Build history of the part. All positions in model axes, mm. Give positions to 0.01 mm unless a question says otherwise; leave off trailing zeros. Order: outer loops, then holes, each group sorted by start corner. A loop starts at its lowest first (then second) coordinate and runs counter-clockwise, first axis right, second up. Notation, with made-up numbers: (-17.5, 28.25) - (-2.5, 28.25) arc R24 cw to (-2.5, 53.25) - close; hole circle Ø3 at (27.25, -5.5). An arc over 180 degrees is marked (long way). One line per item, written item: value.
```python
from build123d import *

# Parameters (mm, degrees)
F0_W       = 47.1339412034
F0_H       = 49.880169332
F1_DEPTH   = 49.1529554129
F1_FACE_W  = 47.1339412034
F1_FACE_H  = 49.880169332
F1_FACE1_W = 47.1339412034
F1_FACE1_H = 49.880169332
F3_R       = 5.08


with BuildPart() as f1:
    # F0 (on Top) → F1 (new body)
    with BuildSketch(Plane.XY):
        with Locations((7.0049632341, -4.9151517451)):
            Rectangle(F0_W, F0_H)
    extrude(amount=F1_DEPTH)

    # F1_face (on face) → F2 section 0
    with BuildSketch(Plane(origin=(7.0049632341, -4.9151517451, 0), x_dir=(1, 0, 0), z_dir=(0, 0, -1))):
        Rectangle(F1_FACE_W, F1_FACE_H)
    # F1_face1 (on face) → F2 section 1
    with BuildSketch(Plane(origin=(7.0049632341, -4.9151517451, 49.1529554129), x_dir=(1, 0, 0), z_dir=(0, 0, 1))):
        Rectangle(F1_FACE1_W, F1_FACE1_H)
    loft()

    # F3
    f3_edges = [f1.edges().sort_by_distance(p)[0] for p in [
        (7.004963, 20.024933, 49.152955),
        (-16.562007, -4.915152, 49.152955),
        (7.004963, 20.024933, 0),
        (-16.562007, -4.915152, 0),
        (-16.562007, 20.024933, 24.576478),
        (7.004963, -29.855236, 49.152955),
        (30.571934, -4.915152, 49.152955),
        (-16.562007, -29.855236, 24.576478),
        (30.571934, -29.855236, 24.576478),
        (7.004963, -29.855236, 0),
        (30.571934, 20.024933, 24.576478),
        (30.571934, -4.915152, 0),
    ]]
    fillet(f3_edges, radius=F3_R)


solid = f1.part
```
(1) Slice it at B-B, the plane x = 27. Give the cut face in (y, z).
Completed:
outline: (-29.63, 5.08) arc R4.85 ccw to (-24.78, 0.23) - (14.94, 0.23) arc R4.85 ccw to (19.8, 5.08) - (19.8, 44.07) arc R4.85 ccw to (14.94, 48.92) - (-24.78, 48.92) arc R4.85 ccw to (-29.63, 44.07) - close
(2) Slice it at A-A, the plane x = -13. Give the cut face in (y, z), and give its area (3 significant figures).
Completed:
outline: (-29.62, 5.08) arc R4.85 ccw to (-24.78, 0.23) - (14.94, 0.23) arc R4.85 ccw to (19.79, 5.08) - (19.79, 44.07) arc R4.85 ccw to (14.94, 48.92) - (-24.78, 48.92) arc R4.85 ccw to (-29.62, 44.07) - close
area: 2,390 mm²
(3) Drill centre lines: line 1 (Y direction, x = -13.5, z = 7); line 2 (Z direction, x = -12, y = -21); line 3 (X direction, y = 6, z = 4.5). Where is each one in solid material? Low to high.
Completed:
line 1: -29.44 to 19.61
line 2: 0.03 to 49.13
line 3: -16.53 to 30.54
